Verification items for this drawing (mm, ordinates from the low corner). A direction names the side the tool comes from. Round coordinates to 2 decimals unless told otherwise and drop trailing zeros. Order: outer loops, then holes, each group sorted by start corner. A loop starts at its lowest first (then second) coordinate and runs counter-clockwise, first axis right, second up. Notation, with made-up numbers: M 22.25,7.25 L 63.25,7.25 A19 cw 63.25,27.25 Z; hole C 16,51 d1. An arc over 180 degrees is marked long. Use CSV: the item, a comma, the result in double quotes. Start each with the question number.
Q1. Gauge pin test, flat end, axial feed: pin 1 Ø6 at (x, z) = (4.5, 4) entering from -Y. Record the tip position at first contact, or that the pin passes through.
Q2. Scan lines: line 1 (X direction, y = 1.85, z = 21.5); line 2 (Z direction, x = 6, y = 2.5). Record each from-to range of solid material in increasing order.
Q3. Mould release check, pull along X, two halves, no side actions. Record for the marked faces 1, 2 and 3: +X half, -X half, draft (parallel to the pull), parting line (faces both ways), or undercut.
Q4. Sectioned sample at C-C (x = 14). Enter the section's corners in (y, z), and give its area (3 significant figures).
Q5. Set-up check for the marked faces 4 and 5: record each of +Z, -Z, +X, -X, +Y, -Y from which the full face is reachable in a straight line by a thin tool's end or side.
Q6. Sectioned sample at A-A (y = 2.1). Enter the section's corners in (x, z), and give its area (3 significant figures).
Q7. Sectioned sample at B-B (x = 18.2). Enter the section's corners in (y, z), and give its area (3 significant figures).
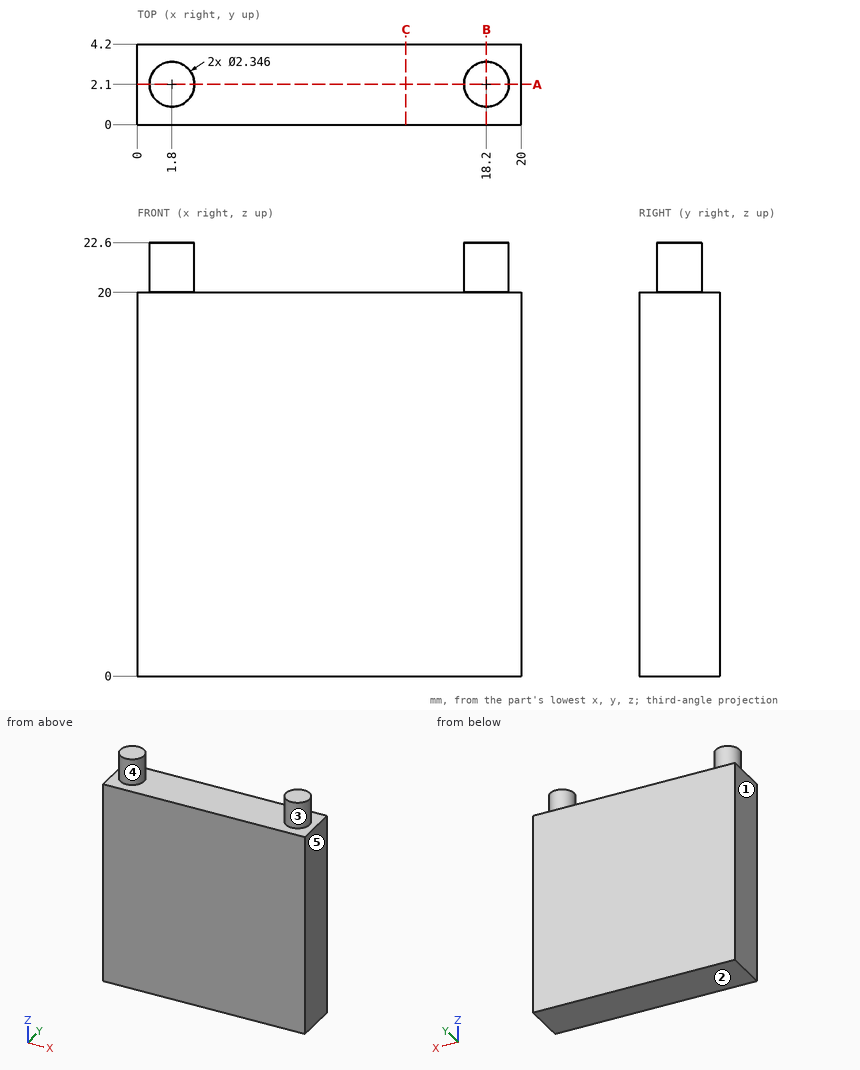
Verdict:
1,pin 1,"stops at y = 0"
2,line 1,"x = 0.65 to 2.95, 17.05 to 19.35"
2,line 2,"z = 0 to 20"
3,face 1,"-X half"
3,face 2,"draft"
3,face 3,"undercut"
4,outline,"M 0,0 L 4.2,0 L 4.2,20 L 0,20 Z"
4,area,"84.0 mm²"
5,face 4,"+Z"
5,face 5,"+Z, -Z, +X, +Y, -Y"
6,outline,"M 0,0 L 20,0 L 20,20 L 19.37,20 L 19.37,22.6 L 17.03,22.6 L 17.03,20 L 2.97,20 L 2.97,22.6 L 0.63,22.6 L 0.63,20 L 0,20 Z"
6,area,"412 mm²"
7,outline,"M 0,0 L 4.2,0 L 4.2,20 L 3.27,20 L 3.27,22.6 L 0.93,22.6 L 0.93,20 L 0,20 Z"
7,area,"90.1 mm²"
